Design review of the part built by this model. Coordinates are the model's own, in mm. Give positions to 0.01 mm unless a question says otherwise; leave off trailing zeros. Order: outer loops, then holes, each group sorted by start corner. A loop starts at its lowest first (then second) coordinate and runs counter-clockwise, first axis right, second up. Notation, with made-up numbers: M 11.25,57 L 55.25,57 A26 cw 55.25,89 Z; hole C 75,-10.75 d6. An arc over 180 degrees is marked long. Answer as a JSON object with one key per item and string values.
from build123d import *

# Parameters (mm, degrees)
SKETCH_1_W          = 199
SKETCH_1_H          = 170
EXTRUDE_1_DEPTH     = 2
SKETCH_2_R          = 2.2
CUT_EXTRUDE_1_DEPTH = 2


with BuildPart() as part:
    # ｽｹｯﾁ1 → ﾎﾞｽ - 押し出し1 (new body)
    with BuildSketch(Plane.XY):
        Rectangle(SKETCH_1_W, SKETCH_1_H)
    extrude(amount=EXTRUDE_1_DEPTH)

    # ｽｹｯﾁ2 → ｶｯﾄ - 押し出し1 (cut)
    with BuildSketch(Plane.XY.offset(2)):
        with Locations((-92, -70)):
            Circle(SKETCH_2_R)
        with Locations((-92, -7.5)):
            Circle(SKETCH_2_R)
        with Locations((-92, 55)):
            Circle(SKETCH_2_R)
        with Locations((92, -70)):
            Circle(SKETCH_2_R)
        with Locations((92, -7.5)):
            Circle(SKETCH_2_R)
        with Locations((92, 55)):
            Circle(SKETCH_2_R)
    extrude(amount=-CUT_EXTRUDE_1_DEPTH, mode=Mode.SUBTRACT)


solid = part.part
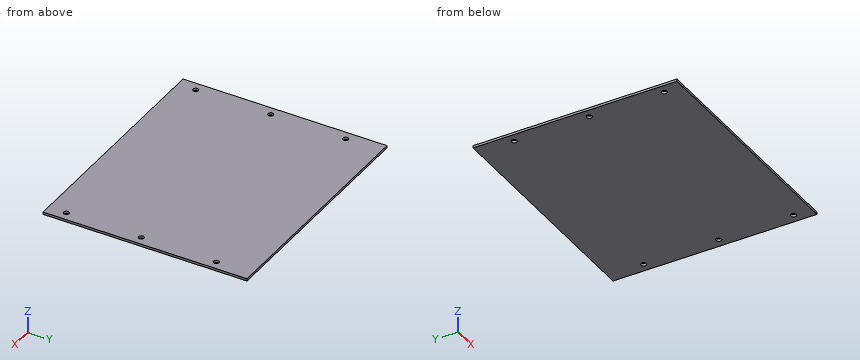
(1) We need section A-A (y = -7.5). Write out the cut boundary in (x, z), plus the area to 3 significant figures.
Checked values:
{"outline": "M -99.5,0 L -94.2,0 L -94.2,2 L -99.5,2 Z; M -89.8,0 L 89.8,0 L 89.8,2 L -89.8,2 Z; M 94.2,0 L 99.5,0 L 99.5,2 L 94.2,2 Z", "area": "380 mm^2"}
(2) To check wall thickness, follow L1, parallel to Y at x = 92, z = 0.8; L2, parallel to X at y = -71.5, z = 1.1; L3, parallel to X at y = -8, z = 1.6. State the ranges of each line that lie inside material, in increasing order. Write a range as from..to.
Checked values:
{"L1": "y = -85..-72.2, -67.8..-9.7, -5.3..52.8, 57.2..85", "L2": "x = -99.5..-93.61, -90.39..90.39, 93.61..99.5", "L3": "x = -99.5..-94.14, -89.86..89.86, 94.14..99.5"}
(3) We need section B-B (x = 92). Write out the cut boundary in (y, z), plus the area to 3 significant figures.
Checked values:
{"outline": "M -85,0 L -72.2,0 L -72.2,2 L -85,2 Z; M -67.8,0 L -9.7,0 L -9.7,2 L -67.8,2 Z; M -5.3,0 L 52.8,0 L 52.8,2 L -5.3,2 Z; M 57.2,0 L 85,0 L 85,2 L 57.2,2 Z", "area": "314 mm^2"}
(4) Insertion check: pin 1 (3.5 mm diameter, centred on x = 92, y = -7.5, fed in from -Z). The pin has a flat end and moves straight along its axis. Give the tip position at first contact, or say it passes through.
Checked values:
{"pin 1": "passes through"}
